Autodesk Inventor part; units mm, degrees
ref_plane "XZ Plane" through (0, 0, 0) normal (0, 1, 0) x (-1, 0, 0)
ref_plane "XY Plane" through (0, 0, 0) normal (0, 0, 1) x (1, 0, 0)
sketch "Эскиз1" plane through (0, 0, 0) normal (0, 1, 0) x (-1, 0, 0)
  circle A0 centre (0, 0) radius 1
  arc A1 (1.9956, 15.1325) -> (-1.9956, 15.1325) centre (0, 15) ccw
  line L0 (1.9956, 15.1325) -> (2.8667, 2.008)
  line L1 (-1.9956, 15.1325) -> (-2.8667, 2.008)
  circle A2 centre (0, 15) radius 0.25
  circle A3 centre (0, 13) radius 0.25
  circle A4 centre (0, 11) radius 0.25
  circle A5 centre (0, 9) radius 0.25
  circle A6 centre (0, 7) radius 0.25
  circle A7 centre (0, 5) radius 0.25
  line L2 (2.8667, 2.008) -> (3, 0) construction
  line L3 (-2.8667, 2.008) -> (-3, 0) construction
  line L4 (-13.6979, 0) -> (13.2438, 0) construction
  arc A8 (-1.9956, -15.1325) -> (1.9956, -15.1325) centre (0, -15) ccw
  line L5 (1.9956, -15.1325) -> (2.8667, -2.008)
  line L6 (-1.9956, -15.1325) -> (-2.8667, -2.008)
  circle A9 centre (0, -15) radius 0.25
  circle A10 centre (0, -13) radius 0.25
  circle A11 centre (0, -11) radius 0.25
  circle A12 centre (0, -9) radius 0.25
  circle A13 centre (0, -7) radius 0.25
  circle A14 centre (0, -5) radius 0.25
  line L7 (2.8667, -2.008) -> (3, 0) construction
  line L8 (-2.8667, -2.008) -> (-3, 0) construction
  arc A15 (7.25, -1) -> (7.25, 1) centre (7.25, 0) ccw
  arc A16 (-7.25, 1) -> (-7.25, -1) centre (-7.25, 0) ccw
  arc A17 (2.8667, -2.008) -> (3.3541, -1) centre (0, 0) ccw
  arc A18 (3.3541, 1) -> (2.8667, 2.008) centre (0, 0) ccw
  arc A19 (-2.8667, 2.008) -> (-3.3541, 1) centre (0, 0) ccw
  arc A20 (-3.3541, -1) -> (-2.8667, -2.008) centre (0, 0) ccw
  line L9 (7.25, 1) -> (3.3541, 1)
  line L10 (-3.3541, 1) -> (-7.25, 1)
  line L11 (7.25, -1) -> (3.3541, -1)
  line L12 (-3.3541, -1) -> (-7.25, -1)
  circle A21 centre (7.25, 0) radius 0.25
  circle A22 centre (-7.25, 0) radius 0.25
  circle A23 centre (-5.25, 0) radius 0.25
  circle A24 centre (5.25, 0) radius 0.25
  dimension "d1" = 2
  dimension "d2" = 3
  dimension "d3" = 3
  dimension "d4" = 15
  dimension "d5" = 2
  dimension "d6" = 0.5
  dimension "d7" = 0.5
  dimension "d8" = 0.5
  dimension "d9" = 0.5
  dimension "d10" = 0.5
  dimension "d11" = 0.5
  dimension "d13" = 2
  dimension "d14" = 2
  dimension "d15" = 2
  dimension "d16" = 2
  dimension "d17" = 2
  dimension "d32" = 2
  dimension "d33" = 2
  dimension "d34" = 14.5
  dimension "d35" = 7.25
  dimension "d36" = 0.5
  dimension "d37" = 0.5
  dimension "d38" = 0.5
  dimension "d39" = 0.5
  dimension "d40" = 2
  dimension "d41" = 2
extrude "Выдавливание1" add sketch "Эскиз1" along normal blind 1.5
sketch "Эскиз2" plane through (0, 1.5, 0) normal (0, 1, 0) x (1, 0, 0)
  arc A0 (2.8667, -2.008) -> (-3.3541, 1) centre (0, 0) ccw
  circle A1 centre (0, 0) radius 1
  circle A2 centre (0, 0) radius 3.5
  point P0 (-2.8667, -2.008)
extrude "Выдавливание2" add sketch "Эскиз2" along normal blind 2.5
sketch "Эскиз3" plane through (0, 4, 0) normal (0, 1, 0) x (1, 0, 0)
  circle A0 centre (0, 0) radius 1
  circle A1 centre (0, 0) radius 2.25
  dimension "d23" = 4.5
extrude "Выдавливание3" cut sketch "Эскиз3" against normal blind 2
sketch "Эскиз4" plane through (0, 0, 0) normal (0, -1, 0) x (1, 0, 0)
  circle A0 centre (0, 0) radius 2.4
  dimension "d29" = 4.8
extrude "Выдавливание4" cut sketch "Эскиз4" against normal blind 1
equation "\"d7\" = d6"
equation "\"d8\" = d6"
equation "\"d9\" = d6"
equation "\"d10\" = d6"
equation "\"d11\" = d6"
properties part number "Arm 3" material "Нейлон 6/6"
Source: CAD feature listing. Evaluate the final solid. Frame: model axes, mm. A direction names the side the tool comes from. Coordinates: 2 decimals unless noted, no trailing zeros. Write each loop counter-clockwise with the first axis right and the second up, starting at its lowest first coordinate (ties: lowest second). Pieces come first, ordered by that corner, then holes. Notation, with made-up numbers: (6, 29.25) -> (30, 29.25) arc R16 ccw to (30, 52.25) -> close; hole circle Ø2 at (49, -32.5). An arc over 180 degrees is marked (long way). Return JSON: item names as keys, results as strings. Group by question number.
1) Section query B-B, the plane x = 4. Return loops of the section in (y, z).
2) Mould query, pull axis Z, two halves, no side actions, for faces 1 (the face through (0, 0, 3)), 2 (the face through (2.425, 0.74, -8.662)), 3 (the face through (1.29, 0.493, 2.024)). Classes: +Z half, -Z half, draft (parallel to the pull), parting line (faces both ways), or undercut.
3) Contact query for flat-ended pins moving along their axis: P1, Ø1.2, axis at x = 5.5, y = 0.5, coming from the -Z side; P2, Ø1.5, axis at x = 6, y = 3.5, coming from the -Z side; P3, Ø1, axis at x = 5, z = 0.5, coming from the +Y side; P4, Ø1.2, axis at x = 4.5, y = 1, coming from the +Z side. Output: stop coordinate, or through.
4) Ray query, line 1 along Z through (x, y) = (0, 3.45); line 2 along Y through (x, z) = (-1, -14.5); line 3 along Z through (x, y) = (1.75, 3.75). Return the intervals inside material, ascending.
5) Set-up query: faces 4 (the face through (5, 1, 1)), 5 (the face through (8.25, 0.74, -0.02)), 6 (the face through (-5, 1, -1)). Return all of +Z, -Z, +X, -X, +Y, -Y with unobstructed straight access to the full face (end or side cutting, diameter ignored); none if empty.
6) Section query A-A, the plane y = 0.45. State how many separate pieces and enclosed holes the cut face has, plus the area to 3 significant figures.
From the geometry:
{
 "1": {"outline": "(0, -1) -> (1.5, -1) -> (1.5, 1) -> (0, 1) -> close"},
 "2": {"face 1": "draft", "face 2": "-Z half", "face 3": "undercut"},
 "3": {"P1": "z = -1", "P2": "through", "P3": "y = 1.5", "P4": "z = 1"},
 "4": {"line 1": "-3.5 to -2.25, 2.25 to 3.5", "line 2": "0 to 1.5", "line 3": "-3.03 to -1.41, 1.41 to 3.03"},
 "5": {"face 4": "+Z, +X, +Y, -Y", "face 5": "+X, +Y, -Y", "face 6": "-Z, -X, +Y, -Y"},
 "6": {"separate pieces": "1", "enclosed holes": "17", "area": "163 mm²"}
}
